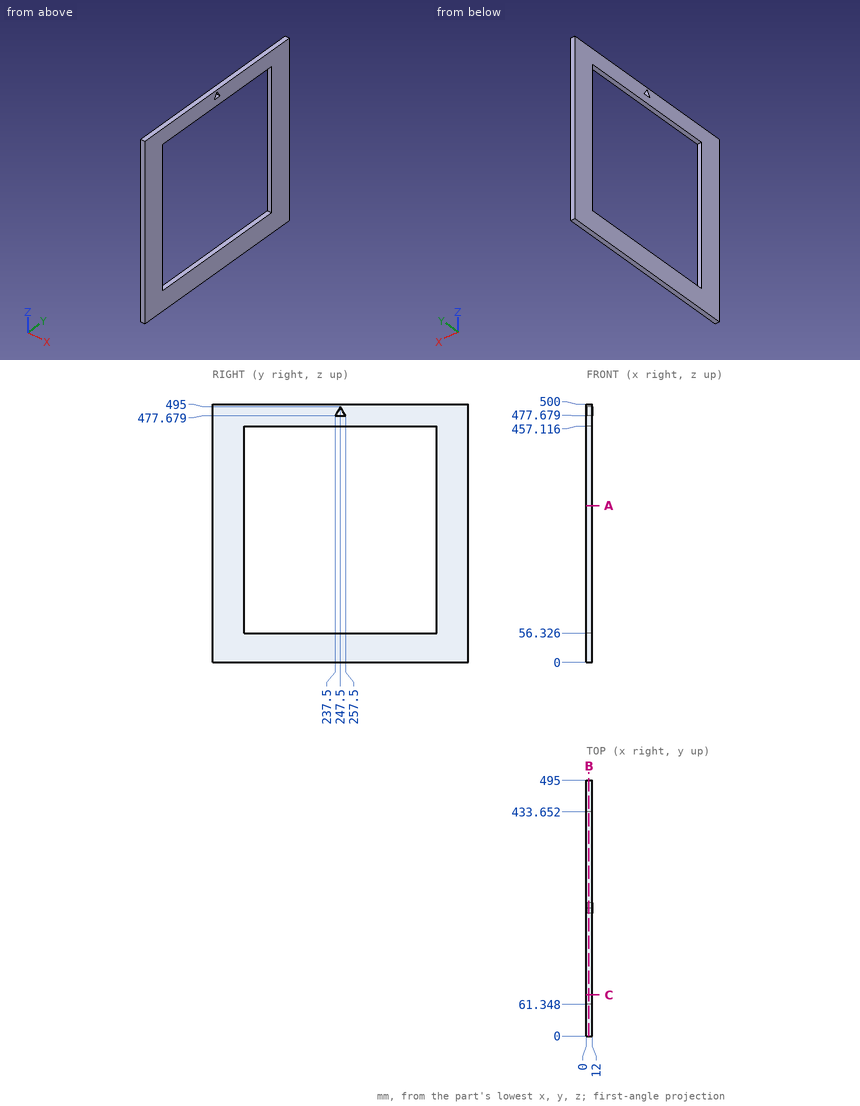
Source: three-view drawing plus pictorial views. Frame: mm from the lowest corner of the part. Give positions to 0.01 mm unless a question says otherwise; leave off trailing zeros. Write each loop counter-clockwise with the first axis right and the second up, starting at its lowest first coordinate (ties: lowest second). Pieces come first, ordered by that corner, then holes.
(1) Cut plane B-B, the plane x = 5. Return loops of the section in (y, z) (1 decimal), then the cut area to 3 significant figures.
(2) Cut plane C-C, the plane y = 79.5. Return loops of the section in (x, z) (1 decimal).
(3) Cut plane A-A, the plane z = 303.5. Return loops of the section in (x, y).
(4) Ray query, line 1 (Z direction, x = 2.5, y = 380.5) (1 decimal); line 2 (Y direction, x = 9, z = 423). Return the intervals inside material, ascending.
Values follow:
1. outline: (0, 0) - (495, 0) - (495, 500) - (0, 500) - close; hole (61.3, 56.3) - (433.7, 56.3) - (433.7, 457.1) - (61.3, 457.1) - close; hole (237.5, 477.7) - (257.5, 477.7) - (247.5, 495) - close
1. area: 98,100 mm2
2. outline: (0, 0) - (12, 0) - (12, 56.3) - (0, 56.3) - close; (0, 457.1) - (12, 457.1) - (12, 500) - (0, 500) - close
3. outline: (0, 0) - (12, 0) - (12, 61.35) - (0, 61.35) - close; (0, 433.65) - (12, 433.65) - (12, 495) - (0, 495) - close
4. line 1: z = 0 to 56.3, 457.1 to 500
4. line 2: y = 0 to 61.35, 433.65 to 495
